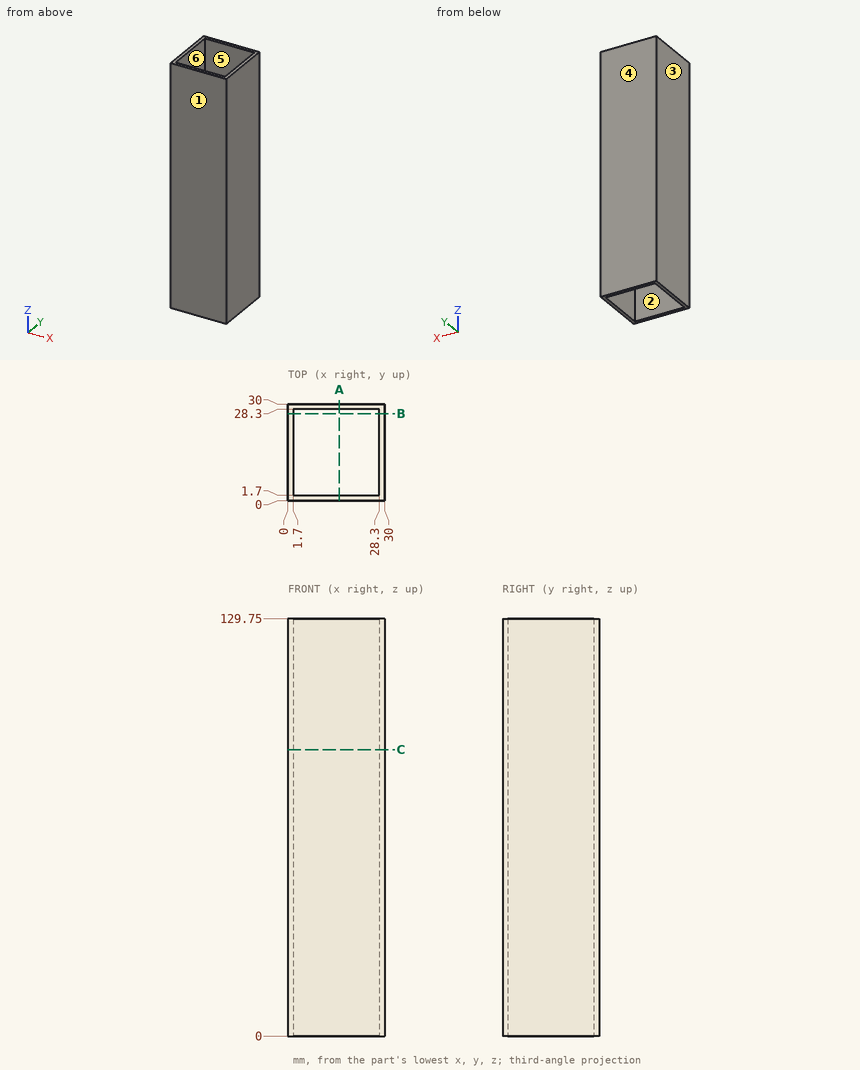
Could you check a few things on this drawing? It's one solid part, dimensions in mm from its lowest x, y, z. A direction names the side the tool comes from. Give positions to 0.01 mm unless a question says otherwise; leave off trailing zeros. Loops run counter-clockwise (first coordinate to the right, second up) from the corner with the lowest first, then second, coordinate; pieces in that order, holes last. Notation, with made-up numbers: M -14.75,62.25 L 37.25,62.25 A14 cw 37.25,70.25 Z; hole C 89,7.25 d11. An arc over 180 degrees is marked long. Answer as a JSON object with one key per item and string values.
Q1. Suppose I cut it at C-C, the plane z = 89. List the corners of the cut face in (x, y) for me, plus the area to 3 significant figures.
Values found:
{"outline": "M 0,0 L 30,0 L 30,30 L 0,30 Z; hole M 1.7,1.7 L 28.3,1.7 L 28.3,28.3 L 1.7,28.3 Z", "area": "192 mm²"}
Q2. Suppose I cut it at A-A, the plane x = 16. List the corners of the cut face in (y, z) for me, plus the area to 3 significant figures.
Values found:
{"outline": "M 0,0 L 1.7,0 L 1.7,129.75 L 0,129.75 Z; M 28.3,0 L 30,0 L 30,129.75 L 28.3,129.75 Z", "area": "441 mm²"}
Q3. If we mould it in two halves opening along Y, with no side actions, what happens to the marked faces 3, 4, 5 and 6? For each: pulls with the +Y half, pulls with the -Y half, needs draft (parallel to the pull), parting line crosses it, or undercut.
Values found:
{"face 3": "needs draft", "face 4": "pulls with the +Y half", "face 5": "undercut", "face 6": "undercut"}
Q4. For the marked faces 1 and 2, which set-ups out of +Z, -Z, +X, -X, +Y, -Y let a thin tool reach every point of the face, with its end or its side?
Values found:
{"face 1": "+Z, -Z, +X, -X, -Y", "face 2": "+Z, -Z"}
Q5. If I drill on probe 1 along X at (y, z) = (18, 58.5), over which ranges is the centre line in solid material (lowest first)? Write a range as [from, to].
Values found:
{"probe 1": "x = [0, 1.7], [28.3, 30]"}
